Can you work these out from the model? Positions are in its coordinate system, mm. Coordinates: 2 decimals unless noted, no trailing zeros. Order: outer loops, then holes, each group sorted by start corner. A loop starts at its lowest first (then second) coordinate and runs counter-clockwise, first axis right, second up. Notation, with made-up numbers: (65, -32.75) -> (105, -32.75) arc R26 ccw to (105, -13.75) -> close; hole circle Ø9 at (-20.75, -13). An arc over 180 degrees is marked (long way). Answer in a Markdown table with one row per item. Add a question column.
1. Imagine slicing it at C-C on y = 1.1. State how many separate pieces and enclosed holes the cut face has, plus the area to 3 significant figures.
2. Imagine slicing it at A-A on x = -25.4. Write out the boundary of the cut face in (y, z), plus the area to 3 significant figures.
3. If I drill on line 1 along Z through (x, y) = (14.5, 0.95); line 2 along X through (y, z) = (0.95, -4); line 3 along X through (y, z) = (1.45, -8.25), over which ranges is the centre line in solid material (lowest first)? Write a range as [from, to].
4. Will these pins go through, and if not, where does the flat tip stop? pin 1 (1 mm diameter, centred on y = 1.5, z = -15.5, fed in from +X); pin 2 (7 mm diameter, centred on x = 39.4, z = -7.51, fed in from -Y); pin 3 (0.6 mm diameter, centred on y = 1.5, z = -16, fed in from -X); pin 4 (0.6 mm diameter, centred on x = 43.5, y = 1, fed in from -Z).
5. Imagine slicing it at B-B on x = 31.5. Write out the boundary of the cut face in (y, z).
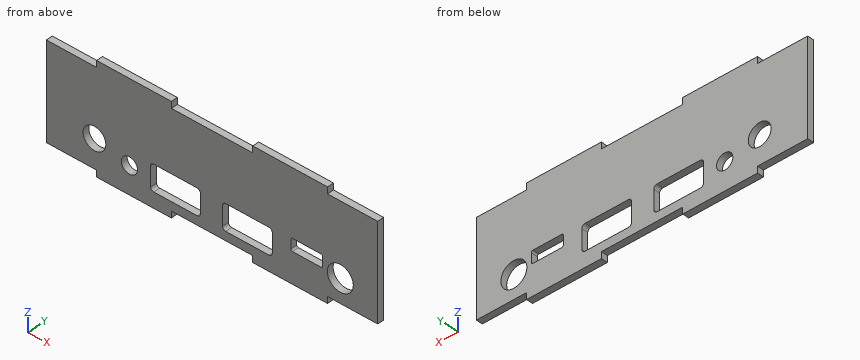
from build123d import *

# Parameters (mm, degrees)
SKETCH_1_W                     = 101.8
SKETCH_1_H                     = 29.5
EXTRUDE_1_DEPTH                = 2
SKETCH_2_W                     = 23
SKETCH_2_H                     = 2
EXTRUDE_2_DEPTH                = 2
SKETCH_3_R                     = 4
CUT_EXTRUDE_1_DEPTH            = 3
SKETCH_4_R                     = 3.5
CUT_EXTRUDE_2_DEPTH            = 3
SKETCH_5_R                     = 2.5
CUT_EXTRUDE_3_DEPTH            = 3
SKETCH_6_W                     = 15.3
SKETCH_6_H                     = 8
CUT_EXTRUDE_4_DEPTH            = 3
FILLET_1_R                     = 1
PATTERN_LINEAR_1_COUNT         = 2
PATTERN_LINEAR_1_PITCH         = 22.1
FILLET_1_OF_PATTERN_LINEAR_1_R = 1
SKETCH_7_W                     = 9.8
SKETCH_7_H                     = 3.8
CUT_EXTRUDE_5_DEPTH            = 3
FILLET_2_R                     = 0.5


with BuildPart() as part:
    # 草图1 → 凸台-拉伸1 (new body)
    with BuildSketch(Plane(origin=(0, 0, 0), x_dir=(1, 0, 0), z_dir=(0, 1, 0))):
        Rectangle(SKETCH_1_W, SKETCH_1_H)
    extrude(amount=EXTRUDE_1_DEPTH)

    # 草图2 → 凸台-拉伸2 (add)
    with BuildSketch(Plane(origin=(0, 2, 0), x_dir=(1, 0, 0), z_dir=(0, 1, 0))):
        with Locations((-24, 15.75)):
            Rectangle(SKETCH_2_W, SKETCH_2_H)
        with Locations((24, 15.75)):
            Rectangle(SKETCH_2_W, SKETCH_2_H)
        with Locations((24, -15.75)):
            Rectangle(SKETCH_2_W, SKETCH_2_H)
        with Locations((-24, -15.75)):
            Rectangle(SKETCH_2_W, SKETCH_2_H)
    extrude(amount=-EXTRUDE_2_DEPTH)

    # 草图3 → 切除-拉伸1 (cut, through all)
    with BuildSketch(Plane(origin=(0, 2, 0), x_dir=(1, 0, 0), z_dir=(0, 1, 0))):
        with Locations((39.4, 7.51)):
            Circle(SKETCH_3_R)
    extrude(amount=-CUT_EXTRUDE_1_DEPTH, mode=Mode.SUBTRACT)

    # 草图4 → 切除-拉伸2 (cut, through all)
    with BuildSketch(Plane(origin=(0, 2, 0), x_dir=(1, 0, 0), z_dir=(0, 1, 0))):
        with Locations((-36.15, 6)):
            Circle(SKETCH_4_R)
    extrude(amount=-CUT_EXTRUDE_2_DEPTH, mode=Mode.SUBTRACT)

    # 草图5 → 切除-拉伸3 (cut, through all)
    with BuildSketch(Plane(origin=(0, 2, 0), x_dir=(1, 0, 0), z_dir=(0, 1, 0))):
        with Locations((-25.4, 8.25)):
            Circle(SKETCH_5_R)
    extrude(amount=-CUT_EXTRUDE_3_DEPTH, mode=Mode.SUBTRACT)

    # 草图6 → 切除-拉伸4 (cut, through all)
    with BuildSketch(Plane(origin=(0, 2, 0), x_dir=(1, 0, 0), z_dir=(0, 1, 0))):
        with Locations((-11.25, 8.05)):
            Rectangle(SKETCH_6_W, SKETCH_6_H)
    cut_extrude_4 = extrude(amount=-CUT_EXTRUDE_4_DEPTH, mode=Mode.SUBTRACT)

    # 圆角1
    fillet_1_edges = [part.edges().sort_by_distance(p)[0] for p in [
        (-18.9, 1, -4.05),
        (-18.9, 1, -12.05),
        (-3.6, 1, -12.05),
        (-3.6, 1, -4.05),
    ]]
    fillet(fillet_1_edges, radius=FILLET_1_R)

    # 阵列(线性)1: 切除-拉伸4 ×2
    with Locations(*[(i * PATTERN_LINEAR_1_PITCH, 0, 0) for i in range(1, PATTERN_LINEAR_1_COUNT)]):
        add(cut_extrude_4, mode=Mode.SUBTRACT)

    # 圆角1 of 阵列(线性)1
    fillet_1_of_pattern_linear_1_edges = [part.edges().sort_by_distance(p)[0] for p in [
        (3.2, 1, -4.05),
        (3.2, 1, -12.05),
        (18.5, 1, -12.05),
        (18.5, 1, -4.05),
    ]]
    fillet(fillet_1_of_pattern_linear_1_edges, radius=FILLET_1_OF_PATTERN_LINEAR_1_R)

    # 草图7 → 切除-拉伸5 (cut, through all)
    with BuildSketch(Plane(origin=(0, 2, 0), x_dir=(1, 0, 0), z_dir=(0, 1, 0))):
        with Locations((29.1, 5.45)):
            Rectangle(SKETCH_7_W, SKETCH_7_H)
    extrude(amount=-CUT_EXTRUDE_5_DEPTH, mode=Mode.SUBTRACT)

    # 圆角2
    fillet_2_edges = [part.edges().sort_by_distance(p)[0] for p in [
        (24.2, 1, -3.55),
        (24.2, 1, -7.35),
        (34, 1, -7.35),
        (34, 1, -3.55),
    ]]
    fillet(fillet_2_edges, radius=FILLET_2_R)


solid = part.part
Answers follow:
| question | item | result |
|---|---|---|
| 1 | separate pieces | 1 |
| 1 | enclosed holes | 6 |
| 1 | area | 2,800 mm² |
| 2 | outline | (0, -16.75) -> (2, -16.75) -> (2, -10.75) -> (0, -10.75) -> close; (0, -5.75) -> (2, -5.75) -> (2, 16.75) -> (0, 16.75) -> close |
| 2 | area | 57.0 mm² |
| 3 | line 1 | z = [-16.75, -12.05], [-4.05, 16.75] |
| 3 | line 2 | x = [-50.9, -39.02], [-33.28, 24.2], [34, 37.48], [41.32, 50.9] |
| 3 | line 3 | x = [-50.9, -38.83], [-33.47, -27.9], [-22.9, -18.9], [-3.6, 3.2], [18.5, 35.47], [43.33, 50.9] |
| 4 | pin 1 | stops at x = 35.5 |
| 4 | pin 2 | passes through |
| 4 | pin 3 | stops at x = -35.5 |
| 4 | pin 4 | stops at z = -14.75 |
| 5 | outline | (0, -16.75) -> (2, -16.75) -> (2, -7.35) -> (0, -7.35) -> close; (0, -3.55) -> (2, -3.55) -> (2, 16.75) -> (0, 16.75) -> close |
